Part model, mm, in its own coordinate system. A direction names the side the tool comes from. Coordinates: 2 decimals unless noted, no trailing zeros. Write each loop counter-clockwise with the first axis right and the second up, starting at its lowest first coordinate (ties: lowest second). Pieces come first, ordered by that corner, then holes. Notation, with made-up numbers: (36, -25) - (67, -25) arc R29 ccw to (67, 9) - close; hole circle Ø1 at (59, -27). An arc over 180 degrees is marked (long way). Use a Markdown table: item, result.
```python
from build123d import *

# Parameters (mm, degrees)
F0_R     = 3.175
F1_DEPTH = 76.2
F2_R     = 6.0833
F3_DEPTH = 4.6482
F4_R     = 4.8895
F5_DEPTH = 4.8768
F6_W     = 1.3843
F6_H     = 1.905
F8_SIZE  = 1.016


with BuildPart() as f1:
    # F0 (on Top) → F1 (new body)
    with BuildSketch(Plane.XY):
        Circle(F0_R)
    extrude(amount=F1_DEPTH)

    # F2 (on face) → F3 (join)
    with BuildSketch(Plane.XY.offset(76.2)):
        Circle(F2_R)
    extrude(amount=F3_DEPTH)

    # F4 (on face) → F5 (join)
    with BuildSketch(Plane.XY.offset(80.8482)):
        Circle(F4_R)
    extrude(amount=F5_DEPTH)

    # F6 (on Front) → F7 (revolve, cut)
    with BuildSketch(Plane.XZ):
        with Locations((4.19735, 83.4771)):
            Rectangle(F6_W, F6_H)
    revolve(axis=Axis((0, 0, 63.428978), (0, 0, -1)), mode=Mode.SUBTRACT)

    # F8
    f8_edges = [f1.edges().sort_by_distance(p)[0] for p in [
        (-4.8895, 0, 85.725),
    ]]
    chamfer(f8_edges, length=F8_SIZE)


solid = f1.part
```
Item 1: Which spindle directions (+Z, -Z, +X, -X, +Y, -Y) get a long thin tool onto all of the face, cutting with end or side? Do faces 4 (the face through (-3.2, 2.1, 84.43)), 5 (the face through (3, -3, 76.2)), 6 (the face through (1, 5, 80.848)), 7 (the face through (-1, 6, 78)). Say none if no direction does.
From the geometry:
| item | result |
|---|---|
| face 4 | none |
| face 5 | -Z |
| face 6 | +Z |
| face 7 | +Z, -Z |
Item 2: Two-plate mould, pull along Z, no slides. Class faces 1 (the face through (0, 0, 85.725)), 2 (the face through (-1.06, -4.773, 81.675)), 3 (the face through (3.343, -1.053, 83.49)): pulls with the +Z half, pulls with the -Z half, needs draft (parallel to the pull), parting line crosses it, or undercut.
From the geometry:
| item | result |
|---|---|
| face 1 | pulls with the +Z half |
| face 2 | needs draft |
| face 3 | undercut |
Item 3: Drop flat-ended pins along their axis: P1, Ø4, axis at y = 2.5, z = 54.5, coming from the +X side; P2, Ø1, axis at y = 2.5, z = 19.5, coming from the +X side; P3, Ø1.5, axis at x = -3.5, z = 39.5, coming from the +Y side. Give the stop position or say it passes through.
From the geometry:
| item | result |
|---|---|
| P1 | x = 3.14 |
| P2 | x = 2.47 |
| P3 | y = 1.59 |
Item 4: Band-saw the part on C-C, the plane z = 23. Give the cut face in (x, y) (3 decimals), then the cut area to 3 significant figures.
From the geometry:
| item | result |
|---|---|
| outline | circle Ø6.35 at (0, 0) |
| area | 31.7 mm^2 |
Item 5: Drill centre lines: probe 1 along Z at (x, y) = (4.25, 0.25); probe 2 along Z at (x, y) = (3.5, -4.25); probe 3 along X at (y, z) = (-0.25, 52.5). Where is each one in solid material? Low to high.
From the geometry:
| item | result |
|---|---|
| probe 1 | 76.2 to 82.52, 84.43 to 85.34 |
| probe 2 | 76.2 to 80.85 |
| probe 3 | -3.17 to 3.17 |
